Geometry check sheet. Reference: the model listing, model coordinates, mm. Face numbers are marked on the shaded views. Give positions to 0.01 mm unless a question says otherwise; leave off trailing zeros. Loops run counter-clockwise (first coordinate to the right, second up) from the corner with the lowest first, then second, coordinate; pieces in that order, holes last. Notation, with made-up numbers: (-33.75, -33.75) -> (4.25, -33.75) arc R20 ccw to (4.25, -20.75) -> close; hole circle Ø4 at (-7, -29). An arc over 180 degrees is marked (long way). Answer as a JSON object with one key per item and string values.
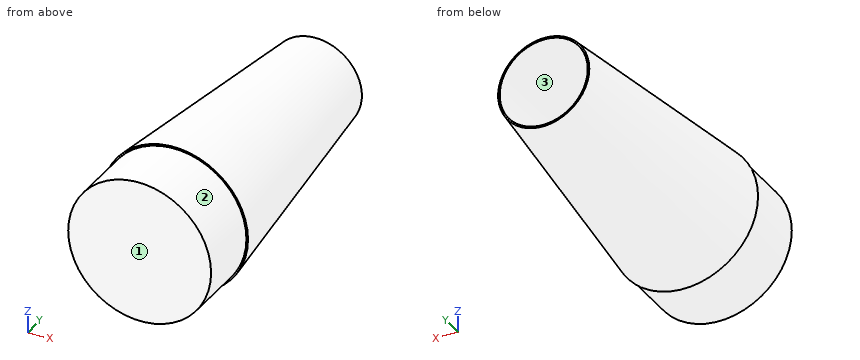
from build123d import *

# Parameters (mm, degrees)
SKETCH2_R          = 52.74818
CUT_EXTRUDE1_DEPTH = 203.2
SKETCH3_OUTSIDE_W  = 267.931
SKETCH3_OUTSIDE_H  = 267.93
SKETCH3_OUTSIDE_R  = 85.6234
CUT_EXTRUDE2_DEPTH = 76.2


with BuildPart() as part:
    # Sketch1 → Revolve1 (revolve)
    with BuildSketch(Plane.XY):
        Polygon((0, 0), (0, 76.2), (32.87522, 381), (87.5284, 381), (87.5284, 0), align=None)
    revolve(axis=Axis((87.5284, 381, 0), (0, -1, 0)))

    # Sketch2 → Cut-Extrude1 (cut)
    with BuildSketch(Plane(origin=(0, 381, 0), x_dir=(1, 0, 0), z_dir=(0, 1, 0))):
        with Locations(Location((87.5284, 0, 0), (0, 0, 180))):
            Circle(SKETCH2_R)
    extrude(amount=-CUT_EXTRUDE1_DEPTH, mode=Mode.SUBTRACT)

    # Sketch3 outside → Cut-Extrude2 (cut)
    with BuildSketch(Plane.XZ):
        with Locations((87.5285, 0)):
            Rectangle(SKETCH3_OUTSIDE_W, SKETCH3_OUTSIDE_H)
        with Locations((87.5284, 0)):
            Circle(SKETCH3_OUTSIDE_R, mode=Mode.SUBTRACT)
    extrude(amount=-CUT_EXTRUDE2_DEPTH, mode=Mode.SUBTRACT)


solid = part.part
1) Depth check by flat-ended pin: P1, Ø1, axis at y = 150, z = 35, coming from the -X side; P2, Ø8, axis at y = 154, z = -47.5, coming from the +X side; P3, Ø8, axis at y = 79, z = 37, coming from the +X side. Enter the tip coordinate at first touch or a pass-through.
Geometry check:
{"P1": "stops at x = 15.82", "P2": "stops at x = 153.69", "P3": "stops at x = 168.34"}
2) Section check B-B on y = 34. Record the cut outline in (x, z).
Geometry check:
{"outline": "circle Ø171.25 at (87.53, 0)"}
3) Material ranges on line 1 along Y through (x, z) = (69, 40.5); line 2 along X through (y, z) = (183, 2.5); line 3 along Z through (x, y) = (62.5, 282.5), recorded low to high. Write a range as from..to.
Geometry check:
{"line 1": "y = 0..177.8", "line 2": "x = 11.56..34.84, 140.22..163.5", "line 3": "z = -60.29..-46.43, 46.43..60.29"}
4) Section check C-C on y = 207. Record the cut outline in (x, z).
Geometry check:
{"outline": "circle Ø146.84 at (87.53, 0); hole circle Ø105.5 at (87.53, 0)"}
5) Section check D-D on y = 274. Record the cut outline in (x, z).
Geometry check:
{"outline": "circle Ø132.39 at (87.53, 0); hole circle Ø105.5 at (87.53, 0)"}
6) Section check A-A on z = 0. Record the cut outline in (x, y) (3 decimals).
Geometry check:
{"outline": "(0, 76.2) -> (1.905, 76.2) -> (1.905, 0) -> (173.152, 0) -> (173.152, 76.2) -> (175.057, 76.2) -> (142.182, 381) -> (140.277, 381) -> (140.277, 177.8) -> (34.78, 177.8) -> (34.78, 381) -> (32.875, 381) -> close"}
7) Draft check along X on the marked faces 1, 2 and 3. Enter one of: pulls with the +X half, pulls with the -X half, needs draft (parallel to the pull), parting line crosses it, or undercut.
Geometry check:
{"face 1": "needs draft", "face 2": "parting line crosses it", "face 3": "undercut"}
